```python
from build123d import *

# Parameters (mm, degrees)
F1_DEPTH  = 16
F2_W      = 6.5
F2_H      = 7
F3_DEPTH  = 6.5
F4_R      = 3.75
F4_R_2    = 2.4
F5_DEPTH  = 10
F6_DEPTH  = 8
F7_R      = 5
F8_DEPTH  = 2.5
F9_DEPTH  = 5
F10_SIZE2 = 2.49999
F10_SIZE  = 2.49999
F11_W     = 9.2321852261
F11_H     = 1
F12_DEPTH = 25


# Not quite as in the source:
# - a fillet or chamfer is up to 0.001 mm smaller than in the source, because OpenCascade refuses the exact size


with BuildPart() as f1:
    # F0 (on Top) → F1 (new body)
    with BuildSketch(Plane.XY):
        with BuildLine():
            Line((2, 13.6), (0, 13.6))
            Line((0, 13.6), (0, 0))
            Line((0, 0), (8.5, 0))
            Line((8.5, 0), (4.7718484698, 2.610479805))
            ThreePointArc((4.7718484698, 2.610479805), (1.425, 4.25), (4.7718484698, 5.889520195))
            Line((4.7718484698, 5.889520195), (8.5, 8.5))
            Line((8.5, 8.5), (2, 8.5))
            Line((2, 8.5), (2, 13.6))
        make_face()
    extrude(amount=F1_DEPTH)

    # F2 (on face) → F3 (cut)
    with BuildSketch(Plane(origin=(0, 8.5, 0), x_dir=(-1, 0, 0), z_dir=(0, 1, 0))):
        with Locations((-5.25, 8)):
            Rectangle(F2_W, F2_H)
    extrude(amount=-F3_DEPTH, mode=Mode.SUBTRACT)

    # F4 (on face) → F5 (join)
    with BuildSketch(Plane(origin=(0, 0, 0), x_dir=(0, -1, 0), z_dir=(-1, 0, 0))):
        with Locations((-6.6, 8)):
            Circle(F4_R)
        with Locations((-6.6, 8)):
            Circle(F4_R_2, mode=Mode.SUBTRACT)
    extrude(amount=F5_DEPTH)

    # F6 (cut): a face of the model
    f6_faces = [f1.faces().sort_by_distance(p)[0] for p in [
        (0, 6.6, 8),
    ]]
    extrude(f6_faces, amount=-F6_DEPTH, mode=Mode.SUBTRACT)

    # F7 (on face) → F8 (join)
    with BuildSketch(Plane(origin=(-10, 0, 0), x_dir=(0, -1, 0), z_dir=(-1, 0, 0))):
        with Locations((-6.6, 8)):
            Circle(F7_R)
    extrude(amount=F8_DEPTH)

    # F9 (cut): a face of the model
    f9_faces = [f1.faces().sort_by_distance(p)[0] for p in [
        (-10, 6.6, 8),
    ]]
    extrude(f9_faces, amount=-F9_DEPTH, mode=Mode.SUBTRACT)

    # F10 (size 2.5 and 2.5 in the source; OpenCascade refuses exactly that, so slightly less here)
    f10_edges = [f1.edges().sort_by_distance(p)[0] for p in [
        (-12.5, 11.6, 8),
    ]]
    chamfer(f10_edges, length=F10_SIZE, length2=F10_SIZE2)

    # F11 (on face) → F12 (cut)
    with BuildSketch(Plane(origin=(0, 13.6, 0), x_dir=(-1, 0, 0), z_dir=(0, 1, 0))):
        with Locations((7.9738140339, 8.1086927094)):
            Rectangle(F11_W, F11_H)
    extrude(amount=-F12_DEPTH, mode=Mode.SUBTRACT)


solid = f1.part
```
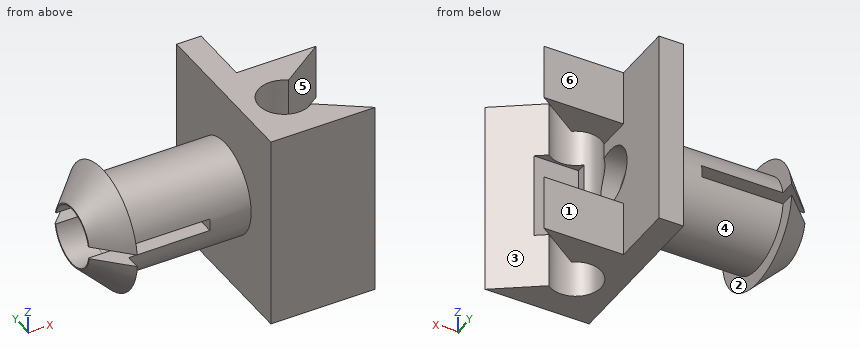
The model under review builds one solid part; all positions refer to its coordinate system, in mm. Face numbers are marked on the shaded views. A direction names the side the tool comes from. Coordinates: 2 decimals unless noted, no trailing zeros. Write each loop counter-clockwise with the first axis right and the second up, starting at its lowest first coordinate (ties: lowest second). Pieces come first, ordered by that corner, then holes. Notation, with made-up numbers: (0, 61) - (15, 61) arc R34 cw to (15, 94) - close; hole circle Ø2 at (-9.75, -8.75). An arc over 180 degrees is marked (long way). Answer in a Markdown table with one row per item. Add a question column.
Q1. Consider section C-C on x = -5.25. Give the boundary of the cut face in (y, z).
Q2. Consider section B-B on z = 2.25. Give the boundary of the cut face in (x, y) (3 decimals), then the cut area to 3 significant figures.
Q3. Consider section D-D on z = 8. Give the boundary of the cut face in (x, y) (3 decimals).
Q4. Consider section A-A on x = 3.5. Give the boundary of the cut face in (y, z) (3 decimals), then the cut area to 4 significant figures.
Q5. Draft analysis for pull direction X (two halves, no side actions). For the marked faces 1, 2 and 3, state which applies: +X half, -X half, draft (parallel to the pull), parting line (faces both ways), or undercut.
Q6. For the marked faces 4, 5 and 6, list the 3-axis set-ups (+Z, -Z, +X, -X, +Y, -Y) from which the entire face can be reached by the end or side of a thin tool; tool diameter is ignored.
Q7. To check wall thickness, follow line 1 along Y through (x, z) = (-2, 8); line 2 along Z through (x, y) = (0.55, 6.6); line 3 along Z through (x, y) = (-3.25, 6.6). State the ranges of each line that lie inside material, in increasing order. Write a range as from..to.
Q8. Clearance check with flat-ended pins moving along their axes: pin 1 (2 mm diameter, centred on x = 5, z = 1.5, fed in from +Y); pin 2 (3 mm diameter, centred on x = -9.5, y = 2.5, fed in from -Z); pin 3 (2 mm diameter, centred on y = 10.5, z = 2.5, fed in from +X). State where each tip first meets the part, or that it passes through.
Answers below:
| question | item | result |
|---|---|---|
| 1 | outline | (2.87, 7.61) arc R3.75 ccw to (10.33, 7.61) - (8.97, 7.61) arc R2.4 cw to (4.23, 7.61) - close; (2.9, 8.61) - (4.28, 8.61) arc R2.4 cw to (8.92, 8.61) - (10.3, 8.61) arc R3.75 ccw to start |
| 2 | outline | (0, 0) - (8.5, 0) - (4.772, 2.61) arc R2.075 cw (long way) to (4.772, 5.89) - (8.5, 8.5) - (2, 8.5) - (2, 13.6) - (0, 13.6) - close |
| 2 | area | 48.8 mm² |
| 3 | outline | (-3.358, 2.85) - (0, 2.85) - (0, 0) - (8.5, 0) - (5.644, 2) - (2, 2) - (2, 2.816) arc R2.075 cw to (1.426, 4.2) - (-3.358, 4.2) - close; (-3.358, 9) - (2, 9) - (2, 13.6) - (0, 13.6) - (0, 10.35) - (-3.358, 10.35) - close |
| 4 | outline | (0, 0) - (2.175, 0) - (2.175, 4.5) - (2, 4.5) - (2, 11.5) - (2.175, 11.5) - (2.175, 16) - (0, 16) - close; (6.325, 0) - (8.5, 0) - (8.5, 4.5) - (6.325, 4.5) - close; (6.325, 11.5) - (8.5, 11.5) - (8.5, 16) - (6.325, 16) - close |
| 4 | area | 53.15 mm² |
| 5 | face 1 | draft |
| 5 | face 2 | undercut |
| 5 | face 3 | +X half |
| 6 | face 4 | none |
| 6 | face 5 | +Z, -Z, +X |
| 6 | face 6 | +Z, -Z, +X, +Y |
| 7 | line 1 | 2.85..4.2, 9..10.35 |
| 7 | line 2 | 0..5.6, 10.4..16 |
| 7 | line 3 | 4.25..5.6, 10.4..11.75 |
| 8 | pin 1 | y = 8.5 |
| 8 | pin 2 | z = 3.78 |
| 8 | pin 3 | x = 2 |
